from build123d import *

# Parameters (mm, degrees)
CROQUIS1_W                   = 884.174
CROQUIS1_H                   = 569.976
BRIDA_BASE1_DEPTH            = 1.524
CROQUIS6_W                   = 3.1242
CROQUIS6_H                   = 6.35
CORTAR_EXTRUIR1_DEPTH        = 526.986119863
BRIDA_START                  = -438.9628
BRIDA_DE_ARISTA1_DEPTH       = 877.9256
BRIDA_START_2                = 6.35
BRIDA_DE_ARISTA1_2_DEPTH     = 557.276
BRIDA_DE_ARISTA1_3_DEPTH     = 877.9256
BRIDA_DE_ARISTA1_4_OUTLINE_W = 0.1524
BRIDA_DE_ARISTA1_4_OUTLINE_H = 1.524
BRIDA_DE_ARISTA1_4_DEPTH     = 0.0762
BRIDA_START_3                = 438.8866
BRIDA_DE_ARISTA1_5_OUTLINE_W = 0.1524
BRIDA_DE_ARISTA1_5_OUTLINE_H = 1.524
BRIDA_DE_ARISTA1_5_DEPTH     = 0.0762
BRIDA_DE_ARISTA1_6_DEPTH     = 557.276
CROQUIS19_R                  = 3.9624
CORTAR_EXTRUIR2_DEPTH        = 527.328773879


# Read off the part's stored shape, not the designer's step: Brida de arista1
# Sheet-metal steps are written as plain solids
with BuildPart() as part:
    # Croquis1 → Brida base1 (new body)
    with BuildSketch(Plane.XY):
        Rectangle(CROQUIS1_W, CROQUIS1_H)
    extrude(amount=-BRIDA_BASE1_DEPTH)

    # Croquis6 → Cortar-Extruir1 (cut, through all)
    with BuildSketch(Plane.XY):
        with Locations((440.5249, 281.813)):
            Rectangle(CROQUIS6_W, CROQUIS6_H)
        with Locations((-440.5249, 281.813)):
            Rectangle(CROQUIS6_W, CROQUIS6_H)
        with Locations((-440.5249, -281.813)):
            Rectangle(CROQUIS6_W, CROQUIS6_H)
        with Locations((440.5249, -281.813)):
            Rectangle(CROQUIS6_W, CROQUIS6_H)
    extrude(amount=-CORTAR_EXTRUIR1_DEPTH, mode=Mode.SUBTRACT)

    # Brida de arista1 outline → Brida de arista1 (add)
    with BuildSketch(Plane.YZ.offset(BRIDA_START)):
        with BuildLine():
            Line((284.988, -19.05), (284.988, -3.048))
            ThreePointArc((284.988, -3.048), (284.884141918, -2.259119551), (284.579645431, -1.524))
            Line((284.579645431, -1.524), (281.94, -1.524))
            ThreePointArc((281.94, -1.524), (283.017630735, -1.970369265), (283.464, -3.048))
            Line((283.464, -3.048), (283.464, -19.05))
            Line((283.464, -19.05), (284.988, -19.05))
        make_face()
        with BuildLine():
            ThreePointArc((-283.464, -3.048), (-283.017630735, -1.970369265), (-281.94, -1.524))
            Line((-281.94, -1.524), (-284.579645431, -1.524))
            ThreePointArc((-284.579645431, -1.524), (-284.884141918, -2.259119551), (-284.988, -3.048))
            Line((-284.988, -3.048), (-284.988, -19.05))
            Line((-284.988, -19.05), (-283.464, -19.05))
            Line((-283.464, -19.05), (-283.464, -3.048))
        make_face()
    extrude(amount=BRIDA_DE_ARISTA1_DEPTH)

    # Brida de arista1 2 outline → Brida de arista1 2 (add)
    with BuildSketch(Plane(origin=(0, 284.988, -1.524), x_dir=(-1, 0, 0), z_dir=(0, -1, 0)).offset(BRIDA_START_2)):
        with BuildLine():
            Line((-440.563, 1.524), (-440.563, 17.526))
            Line((-440.563, 17.526), (-442.087, 17.526))
            Line((-442.087, 17.526), (-442.087, 1.524))
            ThreePointArc((-442.087, 1.524), (-441.983141918, 0.735119551), (-441.678645431, 0))
            Line((-441.678645431, 0), (-439.039, 0))
            ThreePointArc((-439.039, 0), (-440.116630735, 0.446369265), (-440.563, 1.524))
        make_face()
        with BuildLine():
            ThreePointArc((440.563, 1.524), (440.116630735, 0.446369265), (439.039, 0))
            Line((439.039, 0), (441.678645431, 0))
            ThreePointArc((441.678645431, 0), (441.983141918, 0.735119551), (442.087, 1.524))
            Line((442.087, 1.524), (442.087, 17.526))
            Line((442.087, 17.526), (440.563, 17.526))
            Line((440.563, 17.526), (440.563, 1.524))
        make_face()
    extrude(amount=BRIDA_DE_ARISTA1_2_DEPTH)

    # Brida de arista1 3 outline → Brida de arista1 3 (cut)
    with BuildSketch(Plane.YZ.offset(BRIDA_START)):
        with BuildLine():
            ThreePointArc((281.94, 0), (283.464, -0.408354569), (284.579645431, -1.524))
            Line((284.579645431, -1.524), (284.988, -1.524))
            Line((284.988, -1.524), (284.988, 0))
            Line((284.988, 0), (281.94, 0))
        make_face()
        with BuildLine():
            ThreePointArc((-284.579645431, -1.524), (-283.464, -0.408354569), (-281.94, 0))
            Line((-281.94, 0), (-284.988, 0))
            Line((-284.988, 0), (-284.988, -1.524))
            Line((-284.988, -1.524), (-284.579645431, -1.524))
        make_face()
    extrude(amount=BRIDA_DE_ARISTA1_3_DEPTH, mode=Mode.SUBTRACT)

    # Brida de arista1 4 outline → Brida de arista1 4 (cut)
    with BuildSketch(Plane.YZ.offset(BRIDA_START)):
        with Locations((278.7142, -0.762)):
            Rectangle(BRIDA_DE_ARISTA1_4_OUTLINE_W, BRIDA_DE_ARISTA1_4_OUTLINE_H)
        with Locations((-278.7142, -0.762)):
            Rectangle(BRIDA_DE_ARISTA1_4_OUTLINE_W, BRIDA_DE_ARISTA1_4_OUTLINE_H)
    extrude(amount=BRIDA_DE_ARISTA1_4_DEPTH, mode=Mode.SUBTRACT)

    # Brida de arista1 5 outline → Brida de arista1 5 (cut)
    with BuildSketch(Plane.YZ.offset(BRIDA_START_3)):
        with Locations((278.7142, -0.762)):
            Rectangle(BRIDA_DE_ARISTA1_5_OUTLINE_W, BRIDA_DE_ARISTA1_5_OUTLINE_H)
        with Locations((-278.7142, -0.762)):
            Rectangle(BRIDA_DE_ARISTA1_5_OUTLINE_W, BRIDA_DE_ARISTA1_5_OUTLINE_H)
    extrude(amount=BRIDA_DE_ARISTA1_5_DEPTH, mode=Mode.SUBTRACT)

    # Brida de arista1 6 outline → Brida de arista1 6 (cut)
    with BuildSketch(Plane(origin=(0, 284.988, -1.524), x_dir=(-1, 0, 0), z_dir=(0, -1, 0)).offset(BRIDA_START_2)):
        with BuildLine():
            ThreePointArc((-439.039, -1.524), (-440.563, -1.115645431), (-441.678645431, 0))
            Line((-441.678645431, 0), (-442.087, 0))
            Line((-442.087, 0), (-442.087, -1.524))
            Line((-442.087, -1.524), (-439.039, -1.524))
        make_face()
        with BuildLine():
            Line((442.087, 0), (441.678645431, 0))
            ThreePointArc((441.678645431, 0), (440.563, -1.115645431), (439.039, -1.524))
            Line((439.039, -1.524), (442.087, -1.524))
            Line((442.087, -1.524), (442.087, 0))
        make_face()
    extrude(amount=BRIDA_DE_ARISTA1_6_DEPTH, mode=Mode.SUBTRACT)

    # Croquis19 → Cortar-Extruir2 (cut, through all)
    with BuildSketch(Plane.XY):
        with Locations((-433.451, 127)):
            Circle(CROQUIS19_R)
        with Locations((-433.451, -127)):
            Circle(CROQUIS19_R)
        with Locations((433.451, 127)):
            Circle(CROQUIS19_R)
        with Locations((433.451, -127)):
            Circle(CROQUIS19_R)
    extrude(amount=-CORTAR_EXTRUIR2_DEPTH, mode=Mode.SUBTRACT)


solid = part.part
Geometry check sheet. Reference: the model listing, model coordinates, mm. A direction names the side the tool comes from. Round coordinates to 2 decimals unless told otherwise and drop trailing zeros. Loops run counter-clockwise (first coordinate to the right, second up) from the corner with the lowest first, then second, coordinate; pieces in that order, holes last. Notation, with made-up numbers: (78.25, -24) - (127.25, -24) arc R16 ccw to (127.25, -8) - close; hole circle Ø1 at (-27.75, 14). An arc over 180 degrees is marked (long way). One line per question, with ' | ' between items. Start each with the question number.
1. Cross-section at C-C on x = 363.5. Record the cut outline in (y, z).
2. Tool access check on faces 4 (the face through (-6, 4, -1.524)), 5 (the face through (440.563, 4, -11)), 6 (the face through (-6, 283.464, -11)). Record the directions out of +Z, -Z, +X, -X, +Y, -Y that give a thin tool (end or side, any length) a straight path to the whole face; none if there is none.
3. Cross-section at A-A on z = -9.5. Record the cut outline in (x, y).
4. Draft check along X on faces 1 (the face through (-6, -283.464, -11)), 2 (the face through (-440.563, 4, -11)), 3 (the face through (-442.087, 4, -11)). Enter one of: released by +X, released by -X, zero draft, split by the parting line, or undercut.
5. Scan lines: line 1 (X direction, y = -214, z = -4.25); line 2 (Y direction, x = 230, z = -7.25); line 3 (Z direction, x = 268.5, y = -209). Record each from-to range of solid material in increasing order. Write a range as [from, to].
6. Cross-section at B-B on y = 203. Record the cut outline in (x, z), then the cut area to 3 significant figures.
7. Depth check by flat-ended pin: pin 1 (10.5 mm diameter, centred on x = -433.451, y = 127, fed in from -Z); pin 2 (12 mm diameter, centred on x = -119, y = 14, fed in from +Z); pin 3 (3 mm diameter, centred on y = 281, z = -14, fed in from +X); pin 4 (2.5 mm diameter, centred on x = 441, z = -8.5, fed in from -Y). Enter the tip coordinate at first touch or a pass-through.
Taken from the geometry:
1) outline: (-284.99, -19.05) - (-283.46, -19.05) - (-283.46, -3.05) arc R1.52 cw to (-281.94, -1.52) - (281.94, -1.52) arc R1.52 cw to (283.46, -3.05) - (283.46, -19.05) - (284.99, -19.05) - (284.99, -3.05) arc R3.05 ccw to (281.94, 0) - (-281.94, 0) arc R3.05 ccw to (-284.99, -3.05) - close
2) face 4: -Z | face 5: -Z, +Y, -Y | face 6: -Z, +X, -X
3) outline: (-442.09, -278.64) - (-440.56, -278.64) - (-440.56, 278.64) - (-442.09, 278.64) - close; (-438.96, -284.99) - (438.96, -284.99) - (438.96, -283.46) - (-438.96, -283.46) - close; (-438.96, 283.46) - (438.96, 283.46) - (438.96, 284.99) - (-438.96, 284.99) - close; (440.56, -278.64) - (442.09, -278.64) - (442.09, 278.64) - (440.56, 278.64) - close
4) face 1: zero draft | face 2: undercut | face 3: released by -X
5) line 1: [-442.09, -440.56], [440.56, 442.09] | line 2: [-284.99, -283.46], [283.46, 284.99] | line 3: [-1.52, 0]
6) outline: (-442.09, -19.05) - (-440.56, -19.05) - (-440.56, -3.05) arc R1.52 cw to (-439.04, -1.52) - (439.04, -1.52) arc R1.52 cw to (440.56, -3.05) - (440.56, -19.05) - (442.09, -19.05) - (442.09, -3.05) arc R3.05 ccw to (439.04, 0) - (-439.04, 0) arc R3.05 ccw to (-442.09, -3.05) - close | area: 1,400 mm²
7) pin 1: z = -1.52 | pin 2: z = 0 | pin 3: through | pin 4: y = -278.64
